The model under review builds one solid part; all positions refer to its coordinate system, in mm. A direction names the side the tool comes from. Coordinates: 2 decimals unless noted, no trailing zeros. Write each loop counter-clockwise with the first axis right and the second up, starting at its lowest first coordinate (ties: lowest second). Pieces come first, ordered by that corner, then holes. Notation, with made-up numbers: (-32.5, 19) - (18.5, 19) arc R13 ccw to (18.5, 44) - close; hole circle Ø8 at (61, -14.5). An arc over 180 degrees is marked (long way). Answer as CSV lines item,"result". Start each with the question number.
```python
from build123d import *

# Parameters (mm, degrees)
F0_W     = 70
F0_H     = 70
F0_W_2   = 10
F0_H_2   = 10
F0_W_3   = 6
F0_H_3   = 6
F1_DEPTH = 2
F2_DEPTH = 35
F4_DEPTH = 10
F5_W     = 6
F5_H     = 2
F5_H_2   = 6
F6_DEPTH = 7


with BuildPart() as f1:
    # F0 (on Top) → F1 (new body)
    with BuildSketch(Plane.XY):
        Rectangle(F0_W, F0_H)
        Rectangle(F0_W_2, F0_H_2, mode=Mode.SUBTRACT)
        Rectangle(F0_W_2, F0_H_2)
        Rectangle(F0_W_3, F0_H_3, mode=Mode.SUBTRACT)
        Rectangle(F0_W_3, F0_H_3)
    extrude(amount=F1_DEPTH)

    # F0 (on Top) → F2 (join)
    with BuildSketch(Plane.XY):
        Rectangle(F0_W_2, F0_H_2)
        Rectangle(F0_W_3, F0_H_3, mode=Mode.SUBTRACT)
    extrude(amount=F2_DEPTH)

    # F3 (on face) → F4 (join)
    with BuildSketch(Plane.YZ.offset(5)):
        with BuildLine():
            Line((-5, 42), (-5, 35))
            Line((-5, 35), (0, 35))
            Line((0, 35), (0, 36))
            ThreePointArc((0, 36), (-2.5, 38.5), (0, 41))
            Line((0, 41), (0, 42))
            Line((0, 42), (-5, 42))
        make_face()
        with BuildLine():
            Line((0, 36), (0, 35))
            Line((0, 35), (5, 35))
            Line((5, 35), (5, 42))
            Line((5, 42), (0, 42))
            Line((0, 42), (0, 41))
            ThreePointArc((0, 41), (1.767766953, 40.267766953), (2.5, 38.5))
            ThreePointArc((2.5, 38.5), (1.767766953, 36.732233047), (0, 36))
        make_face()
    extrude(amount=-F4_DEPTH)

    # F5 (on face) → F6 (cut)
    with BuildSketch(Plane.XY.offset(42)):
        with Locations((0, -4)):
            Rectangle(F5_W, F5_H)
        Rectangle(F5_W, F5_H_2)
        with Locations((0, 4)):
            Rectangle(F5_W, F5_H)
    extrude(amount=-F6_DEPTH, mode=Mode.SUBTRACT)


solid = f1.part
```
(1) For faces 1 (the flat face through (0, -4, 35)), 2 (the flat face through (-5, 0, 22)), 3 (the flat face through (0, 0, 2)), 4 (the flat face through (5, 0, 22)), 5 (the flat face through (0, 5, 22)), list the 3-axis set-ups (+Z, -Z, +X, -X, +Y, -Y) from which the entire face can be reached by the end or side of a thin tool; tool diameter is ignored.
(2) The part is to be moulded in two halves that separate along Y. For faces 6 (the flat face through (3, 0, 22)), 7 (the flat face through (0, -35, 1)), 8 (the flat face through (0, 0, 0)), 9 (the flat face through (0, 35, 1)), say which applies: released by +Y, released by -Y, zero draft, split by the parting line, or undercut.
(3) For pin 1 (5 mm diameter, centred on x = 1, z = 26.5, fed in from +Y); pin 2 (8 mm diameter, centred on y = -2.5, z = 16.5, fed in from +X); pin 3 (3 mm diameter, centred on x = 5.5, z = 15, fed in from -Y), all flat-tipped, find the tip position at first contact; note any pin that passes through.
(4) Add section A-A on y = 1.5. Give the boundary of the cut face in (x, z).
(5) Add section D-D on x = 7.5. Give the boundary of the cut face in (y, z).
(6) Wall thickness on line 1 (X direction, y = 0.5, z = 10); line 2 (Z direction, x = -28, y = -10): over which ranges is each line inside the solid? List them lowest first.
(7) Add section B-B on z = 25. Give the boundary of the cut face in (x, y).
(8) Add section C-C on z = 37. Give the boundary of the cut face in (x, y), then the cut area to 3 significant figures.
Reported:
1,face 1,"+Z, +Y, -Y"
1,face 2,"+Z, -X, +Y, -Y"
1,face 3,"+Z"
1,face 4,"+Z, +X, +Y, -Y"
1,face 5,"+Z, +X, -X, +Y"
2,face 6,"undercut"
2,face 7,"released by -Y"
2,face 8,"zero draft"
2,face 9,"released by +Y"
3,pin 1,"y = 5"
3,pin 2,"x = 5"
3,pin 3,"y = -5"
4,outline,"(-35, 0) - (35, 0) - (35, 2) - (5, 2) - (5, 36.5) - (3, 36.5) - (3, 2) - (-3, 2) - (-3, 36.5) - (-5, 36.5) - (-5, 2) - (-35, 2) - close; (-5, 40.5) - (-3, 40.5) - (-3, 42) - (-5, 42) - close; (3, 40.5) - (5, 40.5) - (5, 42) - (3, 42) - close"
5,outline,"(-35, 0) - (35, 0) - (35, 2) - (-35, 2) - close"
6,line 1,"-5 to -3, 3 to 5"
6,line 2,"0 to 2"
7,outline,"(-5, -5) - (5, -5) - (5, 5) - (-5, 5) - close; hole (-3, -3) - (3, -3) - (3, 3) - (-3, 3) - close"
8,outline,"(-5, -5) - (-3, -5) - (-3, -2) - (-5, -2) - close; (-5, 2) - (-3, 2) - (-3, 5) - (-5, 5) - close; (3, -5) - (5, -5) - (5, -2) - (3, -2) - close; (3, 2) - (5, 2) - (5, 5) - (3, 5) - close"
8,area,"24.0 mm²"
